from build123d import *

# Parameters (mm, degrees)
SKETCH1_W           = 650
SKETCH1_H           = 30
BOSS_EXTRUDE1_DEPTH = 30
SKETCH2_W           = 20
SKETCH2_H           = 20
BOSS_EXTRUDE2_DEPTH = 15
SKETCH3_W           = 20
SKETCH3_H           = 20
BOSS_EXTRUDE3_DEPTH = 15
SKETCH4_W           = 636.933542964
SKETCH4_H           = 21.079205472
BOSS_EXTRUDE4_DEPTH = 237
SKETCH6_W           = 636.933542964
SKETCH6_H           = 237
SKETCH6_W_2         = 616.933542964
SKETCH6_H_2         = 217
BOSS_EXTRUDE5_DEPTH = 38


with BuildPart() as part:
    # Sketch1 → Boss-Extrude1 (new body)
    with BuildSketch(Plane(origin=(0, 0, 0), x_dir=(1, 0, 0), z_dir=(0, 1, 0))):
        with Locations((-10.201793722, 9.411434978)):
            Rectangle(SKETCH1_W, SKETCH1_H)
    extrude(amount=BOSS_EXTRUDE1_DEPTH)

    # Sketch2 → Boss-Extrude2 (add)
    with BuildSketch(Plane(origin=(314.798206278, 0, 0), x_dir=(0, 0, -1), z_dir=(1, 0, 0))):
        with Locations((9.411434978, 15)):
            Rectangle(SKETCH2_W, SKETCH2_H)
    extrude(amount=BOSS_EXTRUDE2_DEPTH)

    # Sketch3 → Boss-Extrude3 (add)
    with BuildSketch(Plane.ZY.offset(335.201793722)):
        with Locations((-9.411434978, 15)):
            Rectangle(SKETCH3_W, SKETCH3_H)
    extrude(amount=BOSS_EXTRUDE3_DEPTH)

    # Sketch4 → Boss-Extrude4 (add)
    with BuildSketch(Plane.XY.offset(5.588565022)):
        with Locations((-10.201793722, 15)):
            Rectangle(SKETCH4_W, SKETCH4_H)
    extrude(amount=BOSS_EXTRUDE4_DEPTH)

    # Sketch6 → Boss-Extrude5 (add)
    with BuildSketch(Plane.XZ.offset(-4.460397264)):
        with Locations((-10.201793722, 124.088565022)):
            Rectangle(SKETCH6_W, SKETCH6_H)
        with Locations((-10.201793722, 124.088565022)):
            Rectangle(SKETCH6_W_2, SKETCH6_H_2, mode=Mode.SUBTRACT)
    extrude(amount=BOSS_EXTRUDE5_DEPTH)


solid = part.part
Can you work these out from the model? Positions are in its coordinate system, mm. A direction names the side the tool comes from. Round coordinates to 2 decimals unless told otherwise and drop trailing zeros. Loops run counter-clockwise (first coordinate to the right, second up) from the corner with the lowest first, then second, coordinate; pieces in that order, holes last. Notation, with made-up numbers: (58, -7.5) - (81, -7.5) arc R9 cw to (81, 7.5) - close; hole circle Ø5 at (7, 77.5). An arc over 180 degrees is marked (long way). Use CSV: the item, a comma, the result in double quotes. Start each with the question number.
1) For pin 1 Ø4.5 at (x, y) = (320, 12) entering from +Z; pin 2 Ø11.5 at (x, y) = (122, -21.5) entering from -Z; pin 3 Ø16.5 at (x, z) = (-343.5, -11.5) entering from -Y, each with a flat end and sliding along its axis, tell me the tip position at first contact or that it passes through.
2) If we section it at B-B on y = 13.5: Write out the boundary of the cut face in (x, z), plus the area to 3 significant figures.
3) If we section it at D-D on y = -18: Write out the boundary of the cut face in (x, z).
4) Please list where these lines run through material, in increasing order: probe 1 along X at (y, z) = (-22, 197.5); probe 2 along Z at (x, y) = (2, -29); probe 3 along Z at (x, y) = (-219.5, 2.5). Write a range as [from, to].
5) For faces 5 (the flat face through (-343, 15, -19.411)), 6 (the flat face through (-15, -14, 232.589)), 7 (the flat face through (-15, 25.54, 122)), 8 (the flat face through (-343, 25, -10)), which set-ups out of +Z, -Z, +X, -X, +Y, -Y let a thin tool reach every point of the face, with its end or its side?
6) If we section it at A-A on z = 190: Write out the boundary of the cut face in (x, y), plus the area to 3 significant figures.
7) If we section it at C-C on x = 8: Write out the boundary of the cut face in (y, z), plus the area to 3 significant figures.
8) We'd pull the mould along X, two halves only. Please class faces 1 (the flat face through (-318.669, -14, 123)), 2 (the flat face through (-328.669, -4, 122)), 3 (the flat face through (-343, 5, -10)), 4 (the flat face through (329.798, 15, -9)): released by +X, released by -X, zero draft, split by the parting line, or undercut.
Geometry results:
1,pin 1,"stops at z = 0.59"
1,pin 2,"stops at z = 5.59"
1,pin 3,"stops at y = 5"
2,outline,"(-350.2, -19.41) - (-335.2, -19.41) - (-335.2, -24.41) - (314.8, -24.41) - (314.8, -19.41) - (329.8, -19.41) - (329.8, 0.59) - (314.8, 0.59) - (314.8, 5.59) - (308.26, 5.59) - (308.26, 242.59) - (-328.67, 242.59) - (-328.67, 5.59) - (-335.2, 5.59) - (-335.2, 0.59) - (-350.2, 0.59) - close"
2,area,"171,000 mm2"
3,outline,"(-328.67, 5.59) - (308.26, 5.59) - (308.26, 242.59) - (-328.67, 242.59) - close; hole (-318.67, 15.59) - (298.26, 15.59) - (298.26, 232.59) - (-318.67, 232.59) - close"
4,probe 1,"x = [-328.67, -318.67], [298.26, 308.26]"
4,probe 2,"z = [5.59, 15.59], [232.59, 242.59]"
4,probe 3,"z = [-24.41, 15.59], [232.59, 242.59]"
5,face 5,"-Z, -X, +Y, -Y"
5,face 6,"-Y"
5,face 7,"+Z, +X, -X, +Y"
5,face 8,"+Z, -Z, -X, +Y"
6,outline,"(-328.67, -33.54) - (-318.67, -33.54) - (-318.67, 4.46) - (298.26, 4.46) - (298.26, -33.54) - (308.26, -33.54) - (308.26, 25.54) - (-328.67, 25.54) - close"
6,area,"14,200 mm2"
7,outline,"(-33.54, 5.59) - (0, 5.59) - (0, -24.41) - (30, -24.41) - (30, 5.59) - (25.54, 5.59) - (25.54, 242.59) - (-33.54, 242.59) - (-33.54, 232.59) - (4.46, 232.59) - (4.46, 15.59) - (-33.54, 15.59) - close"
7,area,"6,660 mm2"
8,face 1,"undercut"
8,face 2,"released by -X"
8,face 3,"zero draft"
8,face 4,"released by +X"
